Could you check a few things on this model? Use its own coordinates, in mm. Coordinates: 2 decimals unless noted, no trailing zeros. Write each loop counter-clockwise with the first axis right and the second up, starting at its lowest first coordinate (ties: lowest second). Pieces come first, ordered by that corner, then holes. Notation, with made-up numbers: M -9.5,89.25 L 26.5,89.25 A25 ccw 26.5,116.25 Z; hole C 47.5,25.25 d9. An arc over 180 degrees is marked long. Answer as CSV lines item,"result". Start each with the question number.
Item 1: If I drill on line 1 along Y through (x, z) = (29, 0.45); line 2 along Y through (x, z) = (31, 0.7); line 3 along Y through (x, z) = (40.5, 1.1), over which ranges is the centre line in solid material (lowest first)? Write a range as [from, to].
Item 2: Suppose I cut it at A-A, the plane x = 0.5. Write out the boundary of the cut face in (y, z).
Item 3: I'm going to push a flat-ended pin straight in: P1, Ø5, axis at x = 4.5, y = -47.5, coming from the +Z side. Where does the tip first touch, or does it pass through?
Item 4: Suppose I cut it at C-C, the plane z = 0.5. Write out the boundary of the cut face in (x, y), and give its area (3 significant figures).
Item 5: Suppose I cut it at B-B, the plane y = 0.5. Write out the boundary of the cut face in (x, z), and give its area (3 significant figures).
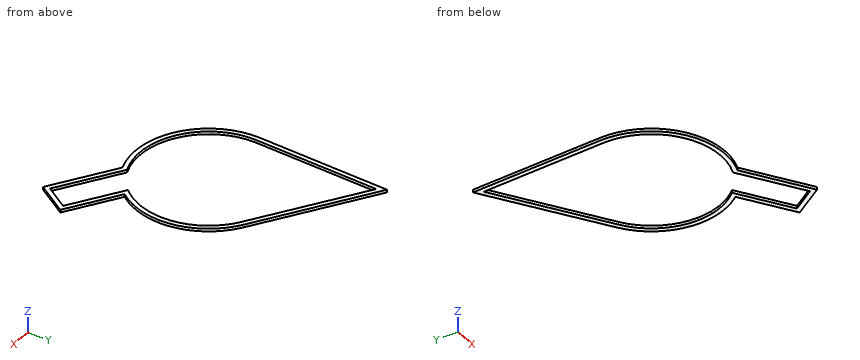
```python
from build123d import *

# Parameters (mm, degrees)
F1_DEPTH = 1.27


with BuildPart() as f1:
    # F0 (on Top) → F1 (new body)
    with BuildSketch(Plane.XY):
        with BuildLine():
            Line((20.811577, 16.726013), (-29.472172, 48.990816))
            Line((-29.472172, 48.990816), (-31.19997, -10.729261))
            ThreePointArc((-31.19997, -10.729261), (-16.887287, -39.323592), (14.856433, -43.17391))
            Line((14.856433, -43.17391), (42.692334, -61.028975))
            Line((42.692334, -61.028975), (51.743443, -46.91837))
            Line((51.743443, -46.91837), (29.216448, -32.468651))
            ThreePointArc((29.216448, -32.468651), (34.516804, -22.683067), (36.349902, -11.70622))
            ThreePointArc((36.349902, -11.70622), (32.211884, 4.494331), (20.811577, 16.726013))
        make_face()
        with BuildLine():
            Line((-29.168819, -10.788025), (-27.544949, 45.339865))
            Line((-27.544949, 45.339865), (19.714212, 15.015803))
            ThreePointArc((19.714212, 15.015803), (30.428787, 3.519862), (34.317901, -11.70622))
            ThreePointArc((34.317901, -11.70622), (34.137361, -15.0873), (33.597794, -18.429929))
            ThreePointArc((33.597794, -18.429929), (33.088689, -20.455162), (32.447555, -22.442549))
            ThreePointArc((32.447555, -22.442549), (31.800913, -24.095469), (31.062915, -25.709672))
            ThreePointArc((31.062915, -25.709672), (30.36012, -27.05728), (29.593639, -28.369712))
            ThreePointArc((29.593639, -28.369712), (27.988575, -30.728623), (26.178225, -32.933916))
            Line((26.178225, -32.933916), (48.935962, -47.531642))
            Line((48.935962, -47.531642), (42.079062, -58.221494))
            Line((42.079062, -58.221494), (15.064719, -40.893409))
            ThreePointArc((15.064719, -40.893409), (-2.08765, -43.11304), (-17.85854, -36.013071))
            ThreePointArc((-17.85854, -36.013071), (-19.098952, -34.914192), (-20.28034, -33.752089))
            ThreePointArc((-20.28034, -33.752089), (-22.513884, -31.173283), (-24.457837, -28.369712))
            ThreePointArc((-24.457837, -28.369712), (-25.224318, -27.05728), (-25.927113, -25.709672))
            ThreePointArc((-25.927113, -25.709672), (-26.665111, -24.095469), (-27.311753, -22.442549))
            ThreePointArc((-27.311753, -22.442549), (-27.955817, -20.444934), (-28.466491, -18.409131))
            ThreePointArc((-28.466491, -18.409131), (-29.04813, -14.619818), (-29.168819, -10.788025))
        make_face(mode=Mode.SUBTRACT)
    extrude(amount=F1_DEPTH)


solid = f1.part
```
Ans:
1,line 1,"y = [-52.25, -49.83], [-34.74, -29.3], [5.88, 9.33]"
1,line 2,"y = [-53.53, -51.11], [-36.03, -33.61], [-29.95, -25.84], [2.42, 6.54]"
1,line 3,"y = [-59.62, -57.21], [-42.12, -39.71]"
2,outline,"M -45.42,0 L -43.39,0 L -43.39,1.27 L -45.42,1.27 Z; M 27.34,0 L 29.76,0 L 29.76,1.27 L 27.34,1.27 Z"
3,P1,"stops at z = 1.27"
4,outline,"M -31.2,-10.73 A33.78 ccw 14.86,-43.17 L 42.69,-61.03 L 51.74,-46.92 L 29.22,-32.47 A33.78 ccw 36.35,-11.71 A33.78 ccw 20.81,16.73 L -29.47,48.99 Z; hole M -29.17,-10.79 A31.75 ccw -28.47,-18.41 A31.75 ccw -27.31,-22.44 A31.75 ccw -25.93,-25.71 A31.75 ccw -24.46,-28.37 A31.75 ccw -20.28,-33.75 A31.75 ccw -17.86,-36.01 A31.75 ccw 15.06,-40.89 L 42.08,-58.22 L 48.94,-47.53 L 26.18,-32.93 A31.75 ccw 29.59,-28.37 A31.75 ccw 31.06,-25.71 A31.75 ccw 32.45,-22.44 A31.75 ccw 33.6,-18.43 A31.75 ccw 34.32,-11.71 A31.75 ccw 19.71,15.02 L -27.54,45.34 Z"
4,area,"632 mm^2"
5,outline,"M -30.88,0 L -28.84,0 L -28.84,1.27 L -30.88,1.27 Z; M 31.88,0 L 34.07,0 L 34.07,1.27 L 31.88,1.27 Z"
5,area,"5.36 mm^2"
